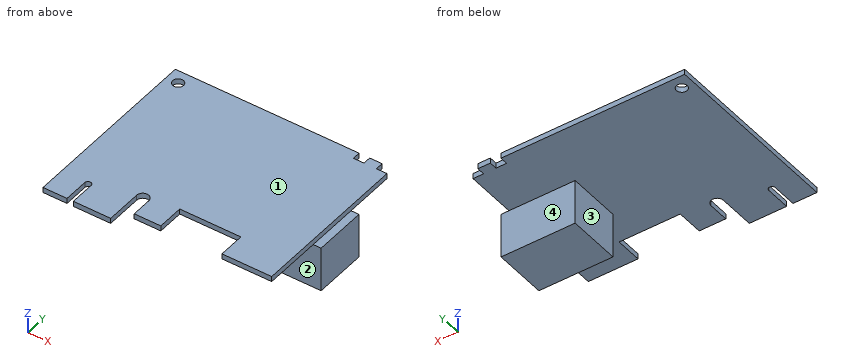
from build123d import *

# Parameters (mm, degrees)
SKETCH2_R           = 1.61925
BOSS_EXTRUDE1_DEPTH = 1.6
SKETCH3_W           = 22.225
SKETCH3_H           = 15.875
BOSS_EXTRUDE2_DEPTH = 13.5


with BuildPart() as part:
    # Sketch2 → Boss-Extrude1 (new body)
    with BuildSketch(Plane.XY):
        with BuildLine():
            Line((0, 0), (7.2, 0))
            Line((7.2, 0), (7.2, 7.45))
            ThreePointArc((7.2, 7.45), (8.15, 8.4), (9.1, 7.45))
            Line((9.1, 7.45), (9.1, 0))
            Line((9.1, 0), (20.3, 0))
            Line((20.3, 0), (20.3, 10.8712))
            ThreePointArc((20.3, 10.8712), (22.1288, 12.7), (23.9576, 10.8712))
            Line((23.9576, 10.8712), (23.9576, 4.7625))
            Line((23.9576, 4.7625), (31.9205, 4.7625))
            Line((31.9205, 4.7625), (31.9205, 12.7))
            Line((31.9205, 12.7), (50.2593, 12.7))
            Line((50.2593, 12.7), (50.2593, 4.7625))
            Line((50.2593, 4.7625), (65.1764, 4.7625))
            Line((65.1764, 4.7625), (65.1764, 53.11875))
            Line((65.1764, 53.11875), (62.0014, 53.11875))
            Line((62.0014, 53.11875), (62.0014, 55.5))
            Line((62.0014, 55.5), (58.2814, 55.5))
            Line((58.2814, 55.5), (58.2814, 53.11875))
            Line((58.2814, 53.11875), (55.1064, 53.11875))
            Line((55.1064, 53.11875), (55.1064, 55.5))
            Line((55.1064, 55.5), (0, 55.5))
            Line((0, 55.5), (0, 0))
        make_face()
        with Locations((3.625, 51.625)):
            Circle(SKETCH2_R, mode=Mode.SUBTRACT)
    extrude(amount=BOSS_EXTRUDE1_DEPTH)

    # Sketch3 → Boss-Extrude2 (add)
    with BuildSketch(Plane(origin=(0, 0, 0), x_dir=(-1, 0, 0), z_dir=(0, 0, -1))):
        with Locations((-56.44515, 30.1)):
            Rectangle(SKETCH3_W, SKETCH3_H)
    extrude(amount=BOSS_EXTRUDE2_DEPTH)


solid = part.part
The listing builds one solid part. Answer for the finished solid, in the listing's coordinates (mm). Face numbers are marked on the shaded views. A direction names the side the tool comes from. Give positions to 0.01 mm unless a question says otherwise; leave off trailing zeros. Loops run counter-clockwise (first coordinate to the right, second up) from the corner with the lowest first, then second, coordinate; pieces in that order, holes last. Notation, with made-up numbers: M 34.5,-39.75 L 46.5,-39.75 A12 ccw 46.5,-16.75 Z; hole C 50,44.5 d3. An arc over 180 degrees is marked long. Answer as CSV lines item,"result".
Item 1: The part is cut by section C-C (z = -2.5). Give the vertices of the cut face in (x, y).
Values follow:
outline,"M 45.33,22.16 L 67.56,22.16 L 67.56,38.04 L 45.33,38.04 Z"
Item 2: The part is cut by section A-A (y = 33). Give the vertices of the cut face in (x, z), and give its area (3 significant figures).
Values follow:
outline,"M 0,0 L 45.33,0 L 45.33,-13.5 L 67.56,-13.5 L 67.56,0 L 65.18,0 L 65.18,1.6 L 0,1.6 Z"
area,"404 mm^2"
Item 3: Given pin 1 Ø1.8 at (x, z) = (56, 1) entering from -Y; pin 2 Ø0.8 at (y, z) = (7, 0.5) entering from +X; pin 3 Ø12 at (x, y) = (12, 29.5) entering from -Z, each flat-ended and moving along its own axis, determine where each tip first touches the part or whether it passes through.
Values follow:
pin 1,"stops at y = 4.76"
pin 2,"stops at x = 65.18"
pin 3,"stops at z = 0"
Item 4: Which of the six approach directions +Z, -Z, +X, -X, +Y, -Y give full straight-line access (tool end or side, diameter ignored) to the marked faces 1, 2, 3 and 4?
Values follow:
face 1,"+Z, +X, -X, +Y, -Y"
face 2,"-Z, +X, -X, -Y"
face 3,"-Z, -X, +Y, -Y"
face 4,"-Z, +X, -X, +Y"
Item 5: The part is cut by section B-B (x = 8.15). Give the vertices of the cut face in (y, z).
Values follow:
outline,"M 8.4,0 L 55.5,0 L 55.5,1.6 L 8.4,1.6 Z"
Item 6: Straight lines are drawn through the part: line 1 along Y through (x, z) = (59.5, -3.25); line 2 along Z through (x, y) = (8.5, 15.5); line 3 along X through (y, z) = (29, -10.5). For each, find the intervals that lie inside material, in ascending order. Write a range as [from, to].
Values follow:
line 1,"y = [22.16, 38.04]"
line 2,"z = [0, 1.6]"
line 3,"x = [45.33, 67.56]"
